Drawing for the job (mm, zero at the part's lowest x, y, z). Give positions to 0.01 mm unless a question says otherwise; leave off trailing zeros. Loops run counter-clockwise (first coordinate to the right, second up) from the corner with the lowest first, then second, coordinate; pieces in that order, holes last. Notation, with made-up numbers: (78, 9.25) - (125, 9.25) arc R23 ccw to (125, 28.25) - close; hole circle Ø8 at (3, 64). An arc over 180 degrees is marked (long way). Return JSON: item names as keys, results as strings. Group by question number.
1) Mould opens along Y. For the marked faces 1, 2 and 3 say: released by +Y, released by -Y, zero draft, split by the parting line, or undercut.
2) Slice it at D-D (y = 7). List the corners of the cut face in (x, z).
3) Drop a flat-ended pin along its axis: pin 1 (3 mm diameter, centred on x = 4.5, y = 4.5, fed in from -Z). Give the stop position or say it passes through.
4) Drill centre lines: probe 1 along Y at (x, z) = (4.5, 0.45); probe 2 along X at (y, z) = (5, 0.4); probe 3 along X at (y, z) = (3, 0.75). Where is each one in solid material? Low to high. Write a range as from..to.
5) Slice it at C-C (z = 0.45). List the corners of the cut face in (x, y), and give its area (3 significant figures).
6) Slice it at A-A (y = 4.5). List the corners of the cut face in (x, z).
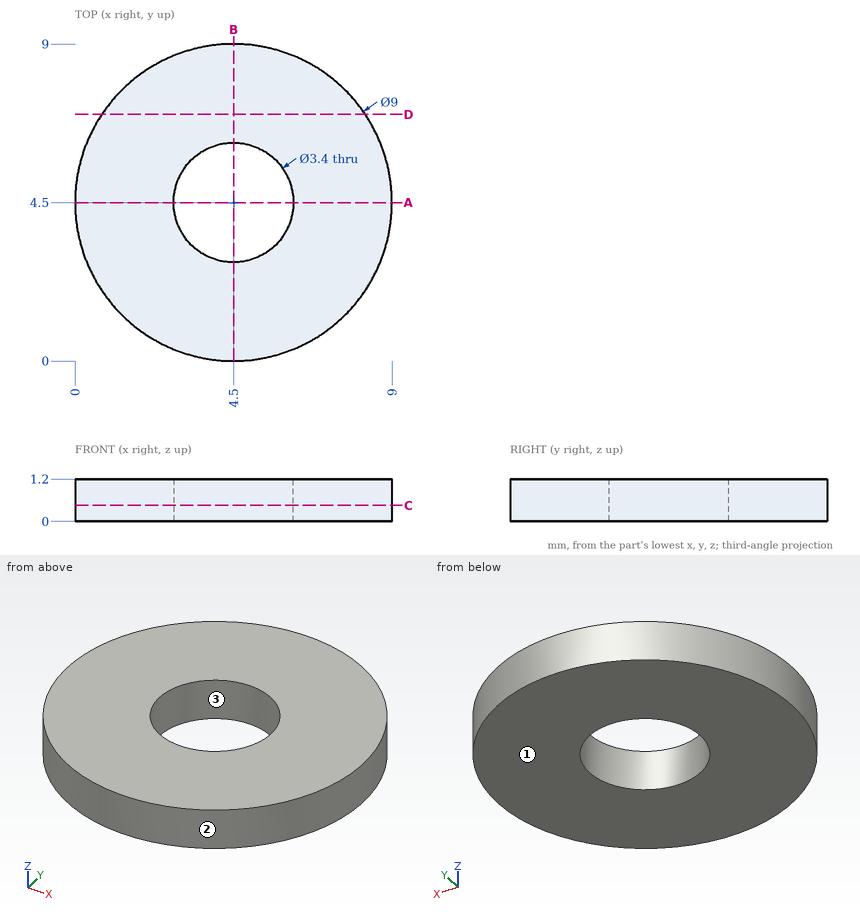
Results:
{
 "1": {"face 1": "zero draft", "face 2": "split by the parting line", "face 3": "undercut"},
 "2": {"outline": "(0.76, 0) - (8.24, 0) - (8.24, 1.2) - (0.76, 1.2) - close"},
 "3": {"pin 1": "through"},
 "4": {"probe 1": "0..2.8, 6.2..9", "probe 2": "0.03..2.88, 6.12..8.97", "probe 3": "0.26..3.7, 5.3..8.74"},
 "5": {"outline": "circle Ø9 at (4.5, 4.5); hole circle Ø3.4 at (4.5, 4.5)", "area": "54.5 mm2"},
 "6": {"outline": "(0, 0) - (2.8, 0) - (2.8, 1.2) - (0, 1.2) - close; (6.2, 0) - (9, 0) - (9, 1.2) - (6.2, 1.2) - close"}
}
